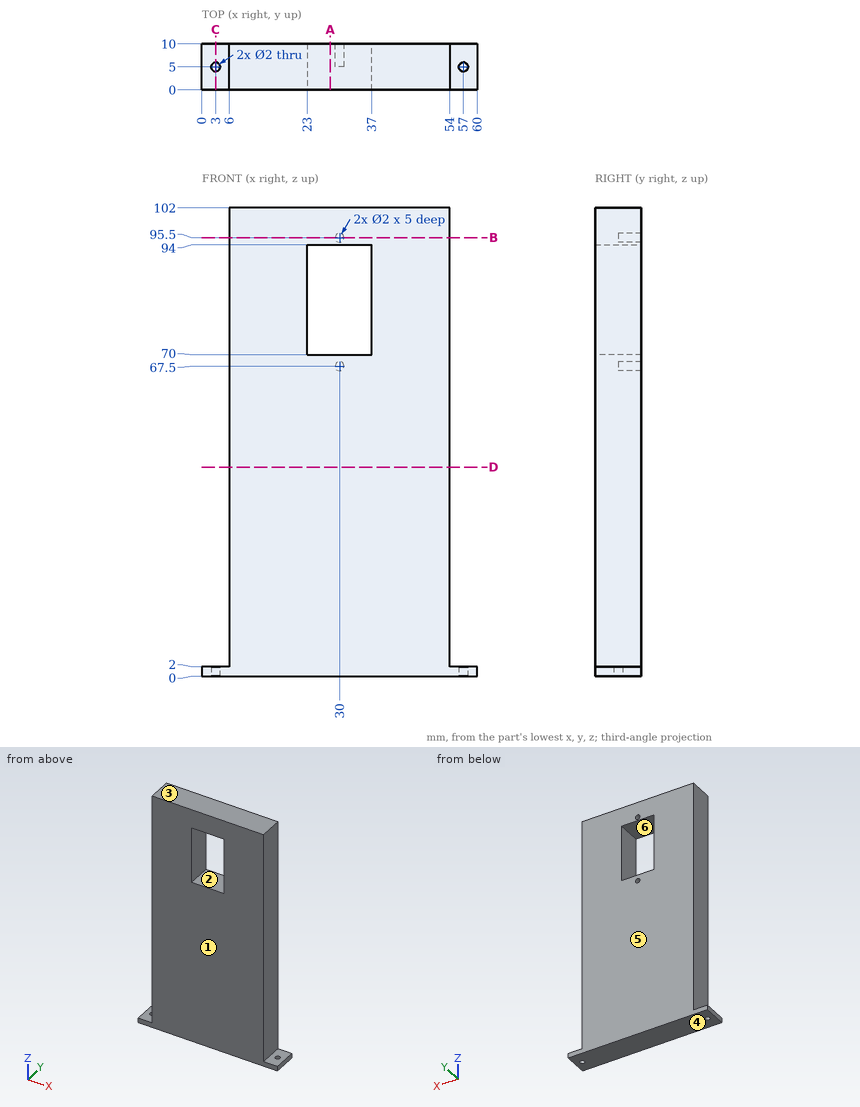
The drawing under review shows one solid part. Ordinate dimensions are in mm from its lowest x, y, z. A direction names the side the tool comes from. Coordinates: 2 decimals unless noted, no trailing zeros. Order: outer loops, then holes, each group sorted by start corner. A loop starts at its lowest first (then second) coordinate and runs counter-clockwise, first axis right, second up. Notation, with made-up numbers: M 76.25,85 L 115.25,85 A9 cw 115.25,99 Z; hole C -28,-24 d2. An arc over 180 degrees is marked long. One line per question, with ' | ' between items.
(1) Add section D-D, the plane z = 45.5. Write out the cut boundary in (x, y).
Geometry results:
outline: M 6,0 L 54,0 L 54,10 L 6,10 Z
(2) Insertion check: pin 1 (6 mm diameter, centred on y = 8, z = 51.5, fed in from +X); pin 2 (0.6 mm diameter, centred on x = 30, z = 67, fed in from +Y); pin 3 (3 mm diameter, centred on y = 3, z = 82.5, fed in from -X). Each pin has a flat end and moves straight along its axis. Give the tip position at first contact, or say it passes through.
Geometry results:
pin 1: stops at x = 54 | pin 2: stops at y = 5 | pin 3: stops at x = 6
(3) Machinability: for the marked faces 5 and 6, which of the approach directions +Z, -Z, +X, -X, +Y, -Y give a long, thin tool a straight path to every point of the face, cutting with its end or side? Answer none if there is none.
Geometry results:
face 5: +Z, -Z, +X, -X, +Y | face 6: +Y, -Y
(4) For probe 1 along Z at (x, y) = (30, 7.7); probe 2 along X at (y, z) = (2.25, 87.5); probe 3 along X at (y, z) = (5, 1.5), list the stretches that pass through material, from the lowest coordinate up. Write a range as from..to.
Geometry results:
probe 1: z = 0..66.5, 68.5..70, 94..94.5, 96.5..102 | probe 2: x = 6..23, 37..54 | probe 3: x = 0..2, 4..56, 58..60
(5) The part is to be moulded in two halves that separate along Z. For the marked faces 1, 2, 3 and 4, say which applies: +Z half, -Z half, draft (parallel to the pull), parting line (faces both ways), or undercut.
Geometry results:
face 1: draft | face 2: undercut | face 3: +Z half | face 4: -Z half
(6) Add section A-A, the plane x = 28. Write out the cut boundary in (y, z), then the cut area to 3 significant figures.
Geometry results:
outline: M 0,0 L 10,0 L 10,70 L 0,70 Z; M 0,94 L 10,94 L 10,102 L 0,102 Z | area: 780 mm²
(7) Add section B-B, the plane z = 95.5. Write out the cut boundary in (x, y).
Geometry results:
outline: M 6,0 L 54,0 L 54,10 L 31,10 L 31,5 L 29,5 L 29,10 L 6,10 Z
(8) Add section C-C, the plane x = 3. Write out the cut boundary in (y, z), then the cut area to 3 significant figures.
Geometry results:
outline: M 0,0 L 4,0 L 4,2 L 0,2 Z; M 6,0 L 10,0 L 10,2 L 6,2 Z | area: 16.0 mm²
